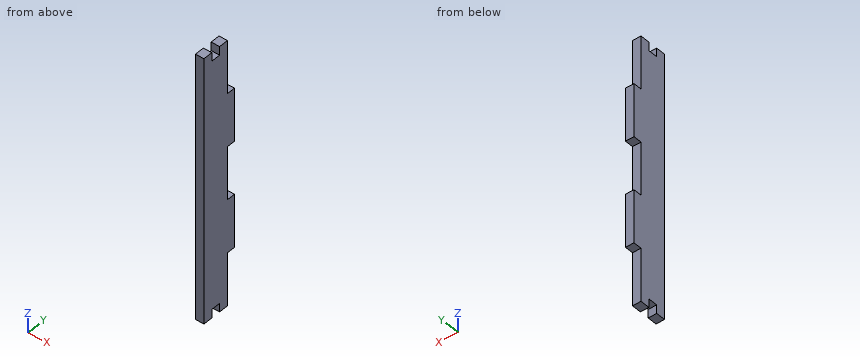
from build123d import *

# Parameters (mm, degrees)
SKETCH1_W               = 415
SKETCH1_H               = 126.5
BOSS_EXTRUDE1_DEPTH     = 6
SKETCH2_W               = 6
SKETCH2_H               = 37.3
BOSS_EXTRUDE2_DEPTH     = 20
SKETCH1_2_W             = 415
SKETCH1_2_H             = 126.5
CUT_EXTRUDE1_DEPTH      = 7
CUT_EXTRUDE1_DEPTH_BACK = 15
SKETCH2_4_W             = 6
SKETCH2_4_H             = 37.3
BOSS_EXTRUDE3_DEPTH     = 6
SKETCH5_W               = 6
SKETCH5_H               = 6.666666666
CUT_EXTRUDE3_DEPTH      = 6


with BuildPart() as part:
    # Sketch1 → Boss-Extrude1 (new body)
    with BuildSketch(Plane(origin=(0, 0, 0), x_dir=(1, 0, 0), z_dir=(0, 1, 0))):
        Rectangle(SKETCH1_W, SKETCH1_H)
    extrude(amount=BOSS_EXTRUDE1_DEPTH)

    # Sketch1<2> → Cut-Extrude1 (cut, two sides)
    with BuildSketch(Plane(origin=(0, 0, 0), x_dir=(1, 0, 0), z_dir=(0, 1, 0))) as cut_extrude1_sk:
        Rectangle(SKETCH1_2_W, SKETCH1_2_H)
    extrude(amount=CUT_EXTRUDE1_DEPTH, mode=Mode.SUBTRACT)
    extrude(cut_extrude1_sk.sketch, amount=-CUT_EXTRUDE1_DEPTH_BACK, mode=Mode.SUBTRACT)


with BuildPart() as body_2:
    # Sketch2 → Boss-Extrude2 (new body)
    with BuildSketch(Plane(origin=(0, 6, 0), x_dir=(1, 0, 0), z_dir=(0, 1, 0))):
        Polygon((-237.5, 55.95), (-231.5, 55.95), (-231.5, 87.25), (-231.5, 93.25), (-237.5, 93.25), align=None)
        with Locations((-234.5, 37.3)):
            Rectangle(SKETCH2_W, SKETCH2_H)
        with Locations((-234.5, 0)):
            Rectangle(SKETCH2_W, SKETCH2_H)
        with Locations((-234.5, -37.3)):
            Rectangle(SKETCH2_W, SKETCH2_H)
        Polygon((-231.5, -93.25), (-231.5, -87.25), (-231.5, -55.95), (-237.5, -55.95), (-237.5, -93.25), align=None)
    extrude(amount=-BOSS_EXTRUDE2_DEPTH)

    # Sketch2<4> → Boss-Extrude3 (add)
    with BuildSketch(Plane(origin=(0, 6, 0), x_dir=(1, 0, 0), z_dir=(0, 1, 0))):
        with Locations((-234.5, -37.3)):
            Rectangle(SKETCH2_4_W, SKETCH2_4_H)
        with Locations((-234.5, 37.3)):
            Rectangle(SKETCH2_4_W, SKETCH2_4_H)
    extrude(amount=BOSS_EXTRUDE3_DEPTH)

    # Sketch5 → Cut-Extrude3 (cut)
    with BuildSketch(Plane.XY.offset(93.25)):
        with Locations((-234.5, -4)):
            Rectangle(SKETCH5_W, SKETCH5_H)
    cut_extrude3 = extrude(amount=-CUT_EXTRUDE3_DEPTH, mode=Mode.SUBTRACT)

    # Mirror3: Cut-Extrude3 across plane
    add(cut_extrude3.mirror(Plane.XY), mode=Mode.SUBTRACT)


solid = body_2.part
Part model, mm, in its own coordinate system. Coordinates: 2 decimals unless noted, no trailing zeros. Order: outer loops, then holes, each group sorted by start corner. A loop starts at its lowest first (then second) coordinate and runs counter-clockwise, first axis right, second up.
(1) Slice it at B-B, the plane x = -236.3. Write the cut outline in (y, z), and give its area (3 significant figures).
Check sheet entries:
outline: (-14, -93.25) - (-7.33, -93.25) - (-7.33, -87.25) - (-0.67, -87.25) - (-0.67, -93.25) - (6, -93.25) - (6, -55.95) - (12, -55.95) - (12, -18.65) - (6, -18.65) - (6, 18.65) - (12, 18.65) - (12, 55.95) - (6, 55.95) - (6, 93.25) - (-0.67, 93.25) - (-0.67, 87.25) - (-7.33, 87.25) - (-7.33, 93.25) - (-14, 93.25) - close
area: 4,100 mm2
(2) Pin check, flat tips, straight feed: pin 1 Ø1.8 at (x, y) = (-234.5, 8) entering from -Z; pin 2 Ø3 at (x, z) = (-235, -2.5) entering from +Y; pin 3 Ø3 at (x, y) = (-234, -3) entering from +Z. Stop position of each tip, or through.
Check sheet entries:
pin 1: stops at z = -55.95
pin 2: stops at y = 6
pin 3: stops at z = 87.25
(3) Slice it at C-C, the plane z = -63. Write the cut outline in (x, y).
Check sheet entries:
outline: (-237.5, -14) - (-231.5, -14) - (-231.5, 6) - (-237.5, 6) - close
(4) Slice it at A-A, the plane y = 8. Write the cut outline in (x, z), and give its area (3 significant figures).
Check sheet entries:
outline: (-237.5, -55.95) - (-231.5, -55.95) - (-231.5, -18.65) - (-237.5, -18.65) - close; (-237.5, 18.65) - (-231.5, 18.65) - (-231.5, 55.95) - (-237.5, 55.95) - close
area: 448 mm2
(5) Probe L1, parallel to Z at x = -232.5, y = 9; L2, parallel to Z at x = -233.7, y = -6; L3, parallel to Y at x = -234.5, z = -12. List the from-to ranges inside material, lowest first.
Check sheet entries:
L1: z = -55.95 to -18.65, 18.65 to 55.95
L2: z = -87.25 to 87.25
L3: y = -14 to 6
(6) Slice it at D-D, the plane y = -5.75. Write the cut outline in (x, z).
Check sheet entries:
outline: (-237.5, -87.25) - (-231.5, -87.25) - (-231.5, 87.25) - (-237.5, 87.25) - close
